Source: CAD feature listing. Evaluate the final solid. Frame: model axes, mm. Face numbers are marked on the shaded views. A direction names the side the tool comes from. Coordinates: 2 decimals unless noted, no trailing zeros. Write each loop counter-clockwise with the first axis right and the second up, starting at its lowest first coordinate (ties: lowest second). Pieces come first, ordered by that corner, then holes. Notation, with made-up numbers: M 68.25,72.25 L 117.25,72.25 A19 ccw 117.25,82.25 Z; hole C 88,16.5 d1. An arc over 180 degrees is marked long. Write item = value, one per line. Start each with the question number.
1. Section query D-D (z = -20.5). Output: boundary loops of the cut face in (x, y) (1 decimal).
2. Access query for the marked faces 5, 6, 7 and 8. Directions: +Z, -Z, +X, -X, +Y, -Y. A direction counts if a zero-diameter tool reaches every point of the face in a straight line with its end or side. Return the directions, or none.
3. Pin query (flat end, axial travel): pin 1 Ø7.5 at (x, y) = (28.5, 15) entering from -Z; pin 2 Ø8 at (x, z) = (19.05, -19.05) entering from -Y (3 decimals); pin 3 Ø21.5 at (x, z) = (30, -24) entering from -Y. Return the tip coordinate at first contact, or that it passes through.
4. Line query: line 1 along Y through (x, z) = (6, -19.5); line 2 along X through (y, z) = (16, -35); line 3 along Z through (x, y) = (28, 22). Output: solid intervals per line, ascending.
5. Section query C-C (z = -10.5). Output: boundary loops of the cut face in (x, y), then the cut area to 3 significant figures.
6. Section query B-B (x = 10). Output: boundary loops of the cut face in (y, z).
7. Pull-direction query (Z, two-part tool) for the marked faces 1, 2, 3 and 4; classes: pulls with the +Z half, pulls with the -Z half, needs draft (parallel to the pull), parting line crosses it, or undercut.
8. Section query A-A (y = 29.5). Output: boundary loops of the cut face in (x, z), then the cut area to 3 significant figures.
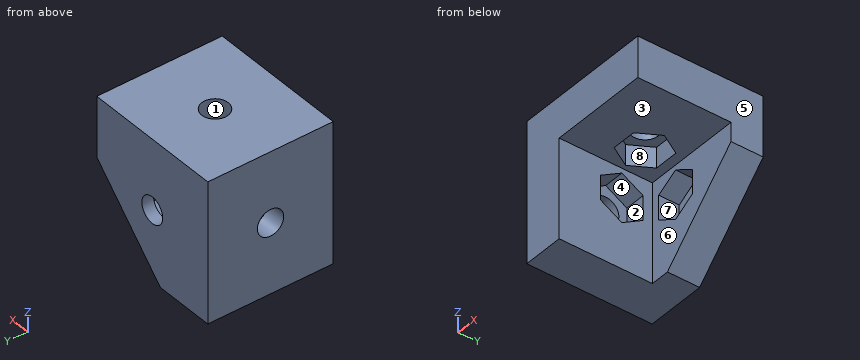
```python
from build123d import *

# Parameters (mm, degrees)
SKETCH1_W                    = 38.1
SKETCH1_H                    = 38.1
MAIN_BODY_DEPTH              = 34
SKETCH3_R                    = 3.571875
F_9_32_RIGHT_RAIL_DEPTH      = 1
F_9_32_RIGHT_RAIL_DEPTH_BACK = 5.55625
SKETCH4_R                    = 3.571875
F_9_32_LEFT_RAIL_DEPTH       = 5.55625
SKETCH8_R                    = 3.571875
F_9_32_TOPPER_DEPTH          = 1
F_9_32_TOPPER_DEPTH_BACK     = 10
HEX_START                    = -5.55625
HEX_HOLE_RIGHT_DEPTH         = 32.54375
HEX_HOLE_LEFT_DEPTH          = 32.54375
INNER_START                  = -17.4625
SKETCH13_W                   = 26.9875
SKETCH13_H                   = 26.9875
INNER_CAVITY_DEPTH           = 8.73125
INNER_CAVITY_DEPTH_BACK      = 22.754687
HEX_START_2                  = -17
HEX_HOLE_TOP_DEPTH           = 13.825
TOP_CORNER_REACH             = 36


with BuildPart() as part:
    # Sketch1 → Main Body (new body)
    with BuildSketch(Plane(origin=(0, 0, 0), x_dir=(1, 0, 0), z_dir=(0, 1, 0))):
        with Locations((19.05, 19.05)):
            Rectangle(SKETCH1_W, SKETCH1_H)
    extrude(amount=MAIN_BODY_DEPTH)

    # Sketch3 → 9/32 Right Rail (cut, two sides)
    with BuildSketch(Plane.XY) as f_9_32_right_rail_sk:
        with Locations((19.05, 17)):
            Circle(SKETCH3_R)
    extrude(amount=F_9_32_RIGHT_RAIL_DEPTH, mode=Mode.SUBTRACT)
    extrude(f_9_32_right_rail_sk.sketch, amount=-F_9_32_RIGHT_RAIL_DEPTH_BACK, mode=Mode.SUBTRACT)

    # Sketch4 → 9/32 Left Rail (cut)
    with BuildSketch(Plane.ZY):
        with Locations((-19.05, 17)):
            Circle(SKETCH4_R)
    extrude(amount=-F_9_32_LEFT_RAIL_DEPTH, mode=Mode.SUBTRACT)

    # Sketch8 → 9/32 Topper (cut, two sides)
    with BuildSketch(Plane(origin=(0, 34, 0), x_dir=(1, 0, 0), z_dir=(0, 1, 0))) as f_9_32_topper_sk:
        with Locations((19.05, 19.05)):
            Circle(SKETCH8_R)
    extrude(amount=F_9_32_TOPPER_DEPTH, mode=Mode.SUBTRACT)
    extrude(f_9_32_topper_sk.sketch, amount=-F_9_32_TOPPER_DEPTH_BACK, mode=Mode.SUBTRACT)

    # Sketch9 → Hex Hole Right (cut)
    with BuildSketch(Plane.ZY.offset(HEX_START)):
        Polygon((-22.372470377, 22.7546875), (-25.694940754, 17), (-22.372470377, 11.2453125), (-15.727529623, 11.2453125), (-12.405059246, 17), (-15.727529623, 22.7546875), align=None)
    extrude(amount=-HEX_HOLE_RIGHT_DEPTH, mode=Mode.SUBTRACT)

    # Sketch10 → Hex Hole Left (cut)
    with BuildSketch(Plane.XY.offset(HEX_START)):
        Polygon((15.727529623, 22.7546875), (12.405059246, 17), (15.727529623, 11.2453125), (22.372470377, 11.2453125), (25.694940754, 17), (22.372470377, 22.7546875), align=None)
    extrude(amount=-HEX_HOLE_LEFT_DEPTH, mode=Mode.SUBTRACT)

    # Sketch13 → Inner Cavity (cut, two sides)
    with BuildSketch(Plane(origin=(0, 34, 0), x_dir=(1, 0, 0), z_dir=(0, 1, 0)).offset(INNER_START)) as inner_cavity_sk:
        with Locations((24.60625, 24.60625)):
            Rectangle(SKETCH13_W, SKETCH13_H)
    extrude(amount=INNER_CAVITY_DEPTH, mode=Mode.SUBTRACT)
    extrude(inner_cavity_sk.sketch, amount=-INNER_CAVITY_DEPTH_BACK, mode=Mode.SUBTRACT)

    # Sketch14 → Hex Hole Top (cut)
    with BuildSketch(Plane(origin=(0, 34, 0), x_dir=(1, 0, 0), z_dir=(0, 1, 0)).offset(HEX_START_2)):
        Polygon((24.8046875, 22.372470377), (19.05, 25.694940754), (13.2953125, 22.372470377), (13.2953125, 15.727529623), (19.05, 12.405059246), (24.8046875, 15.727529623), align=None)
    extrude(amount=HEX_HOLE_TOP_DEPTH, mode=Mode.SUBTRACT)

    # Sketch16 → Top Corner (cut, up to next)
    with BuildSketch(Plane(origin=(0, 34, 0), x_dir=(1, 0, 0), z_dir=(0, 1, 0)), mode=Mode.PRIVATE) as top_corner_sk1:
        Polygon((38.1, 38.1), (16.276714219, 38.1), (38.1, 16.276714219), align=None)
    top_corner_tool1 = extrude(top_corner_sk1.sketch, amount=-TOP_CORNER_REACH, mode=Mode.PRIVATE) & part.part
    add(top_corner_tool1.solids().sort_by_distance((30.825571, 34, -30.825571))[0], mode=Mode.SUBTRACT)


solid = part.part
```
Results are:
q1.outline = M 0,0 L 11.1,0 L 11.1,11.2 L 5.6,11.2 L 5.6,13.7 L 0,13.7 Z; M 0,20.3 L 5.6,20.3 L 5.6,22.8 L 11.1,22.8 L 11.1,25.3 L 13.3,25.3 L 13.3,30.8 L 15.8,30.8 L 15.8,34 L 0,34 Z; M 22.3,30.8 L 24.8,30.8 L 24.8,25.3 L 33.9,25.3 L 33.9,34 L 22.3,34 Z
q2.face_5 = +Z, -Z, +X, +Y, -Y
q2.face_6 = -Z, +X, -Y
q2.face_7 = -Y
q2.face_8 = -Z
q3.pin_1 = -11.11
q3.pin_2 = 30.825
q3.pin_3 = 25.27
q4.line_1 = 0 to 11.25, 22.75 to 34
q4.line_2 = 0 to 11.11
q4.line_3 = -11.11 to 0
q5.outline = M 0,0 L 38.1,0 L 38.1,34 L 0,34 Z; hole M 12.41,17 L 15.73,11.25 L 22.37,11.25 L 25.69,17 L 22.37,22.75 L 15.73,22.75 Z
q5.area = 1,180 mm^2
q6.outline = M 0,-38.1 L 34,-38.1 L 34,0 L 0,0 Z; hole M 11.25,-22.37 L 17,-25.69 L 22.75,-22.37 L 22.75,-15.73 L 17,-12.41 L 11.25,-15.73 Z
q7.face_1 = needs draft
q7.face_2 = undercut
q7.face_3 = pulls with the -Z half
q7.face_4 = undercut
q8.outline = M 0,-38.1 L 16.28,-38.1 L 38.1,-16.28 L 38.1,0 L 0,0 Z; hole M 13.3,-22.37 L 19.05,-25.69 L 24.8,-22.37 L 24.8,-15.73 L 19.05,-12.41 L 13.3,-15.73 Z
q8.area = 1,100 mm^2
